Geometry check sheet. Reference: the model listing, model coordinates, mm. Face numbers are marked on the shaded views. A direction names the side the tool comes from. Round coordinates to 2 decimals unless told otherwise and drop trailing zeros. Order: outer loops, then holes, each group sorted by start corner. A loop starts at its lowest first (then second) coordinate and runs counter-clockwise, first axis right, second up. Notation, with made-up numbers: (68.25, -34.75) - (104.25, -34.75) arc R25 ccw to (104.25, -1.75) - close; hole circle Ø1 at (-22.75, -1). An arc over 180 degrees is marked (long way). One line per question, with ' | ' between items. Start each with the question number.
Q1. Sectioned sample at D-D, the plane z = -2.25. Enter the section's corners in (x, y) (3 decimals), then the cut area to 3 significant figures.
Q2. Sectioned sample at C-C, the plane y = 8.75. Enter the section's corners in (x, z).
Q3. Sectioned sample at A-A, the plane z = 4. Enter the section's corners in (x, y) (3 decimals), then the cut area to 3 significant figures.
Q4. Tool access check on the marked faces 1, 2, 3, 4 and 5. Record the directions out of +Z, -Z, +X, -X, +Y, -Y that give a thin tool (end or side, any length) a straight path to the whole face; none if there is none.
Q5. Material ranges on line 1 along Y through (x, z) = (11.1, 1.25) (3 decimals); line 2 along X through (y, z) = (4.5, 1.25); line 3 along X through (y, z) = (3.75, 4.5), recorded low to high.
Q6. Sectioned sample at B-B, the plane x = 11.1. Enter the section's corners in (y, z) (3 decimals).
Q7. Mould release check, pull along X, two halves, no side actions. Record for the marked faces 6, 7 and 8: +X half, -X half, draft (parallel to the pull), parting line (faces both ways), or undercut.
Q8. Gauge pin test, flat ends, axial feed: P1, Ø2.5, axis at y = 4.5, z = -4, coming from the -X side; P2, Ø3, axis at x = 22.5, y = 4, coming from the -Z side; P3, Ø1.3, axis at x = 24.5, z = -7, coming from the +Y side (3 decimals); P4, Ø3, axis at y = 4.5, z = 6, coming from the -X side. Record the tip position at first contact, or that the pin passes through.
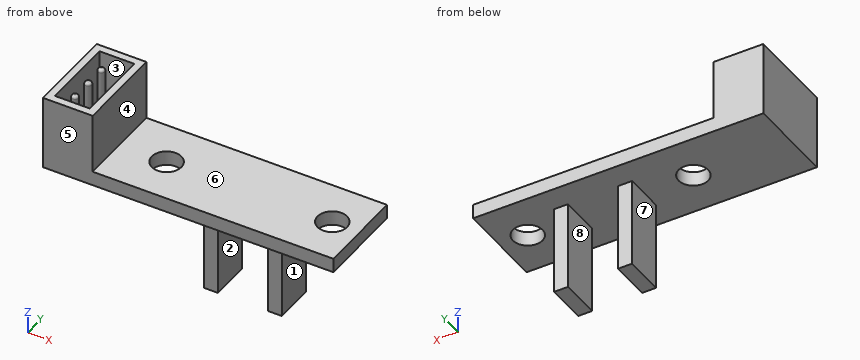
```python
from build123d import *

# Parameters (mm, degrees)
SKETCH_1_W          = 33.3
SKETCH_1_H          = 10.25
EXTRUDE_1_DEPTH     = 1.66
SKETCH_2_W          = 5.7
SKETCH_2_H          = 10.25
EXTRUDE_3_DEPTH     = 6.89
SKETCH_3_W          = 4
SKETCH_3_H          = 8.5
CUT_EXTRUDE_1_DEPTH = 6.05
SKETCH_4_R          = 0.4
EXTRUDE_4_DEPTH     = 5.5
FILLET_1_R          = 0.3
SKETCH_5_R          = 1.7
CUT_EXTRUDE_2_DEPTH = 36.516539809
SKETCH_6_W          = 1.6
SKETCH_6_H          = 4.6
EXTRUDE_5_DEPTH     = 10.19


with BuildPart() as part:
    # Эскиз1 → Бобышка-Вытянуть1 (new body)
    with BuildSketch(Plane.XY):
        with Locations((16.65, 5.125)):
            Rectangle(SKETCH_1_W, SKETCH_1_H)
    extrude(amount=EXTRUDE_1_DEPTH)

    # Эскиз2 → Бобышка-Вытянуть3 (add)
    with BuildSketch(Plane.XY.offset(1.66)):
        with Locations((2.85, 5.125)):
            Rectangle(SKETCH_2_W, SKETCH_2_H)
    extrude(amount=EXTRUDE_3_DEPTH)

    # Эскиз3 → Вырез-Вытянуть1 (cut)
    with BuildSketch(Plane.XY.offset(8.55)):
        with Locations((2.85, 5.125)):
            Rectangle(SKETCH_3_W, SKETCH_3_H)
    extrude(amount=-CUT_EXTRUDE_1_DEPTH, mode=Mode.SUBTRACT)

    # Эскиз4 → Бобышка-Вытянуть4 (add)
    with BuildSketch(Plane.XY.offset(2.5)):
        with Locations((2.050760191, 5.231038637)):
            Circle(SKETCH_4_R)
        with Locations((2.050760191, 7.741038637)):
            Circle(SKETCH_4_R)
        with Locations((2.050760191, 2.721038637)):
            Circle(SKETCH_4_R)
    extrude(amount=EXTRUDE_4_DEPTH)

    # Скругление1
    fillet_1_edges = [part.edges().sort_by_distance(p)[0] for p in [
        (1.650760191, 5.231038637, 8),
        (1.650760191, 7.741038637, 8),
        (1.650760191, 2.721038637, 8),
    ]]
    fillet(fillet_1_edges, radius=FILLET_1_R)

    # Эскиз5 → Вырез-Вытянуть2 (cut, through all)
    with BuildSketch(Plane.XY.offset(1.66)):
        with Locations((11.1, 5.125)):
            Circle(SKETCH_5_R)
        with Locations((30.1, 5.125)):
            Circle(SKETCH_5_R)
    extrude(amount=-CUT_EXTRUDE_2_DEPTH, mode=Mode.SUBTRACT)

    # Эскиз6 → Бобышка-Вытянуть5 (add)
    with BuildSketch(Plane(origin=(0, 0, 0), x_dir=(-1, 0, 0), z_dir=(0, 0, -1))):
        with Locations((-24.9, 5.125)):
            Rectangle(SKETCH_6_W, SKETCH_6_H)
        with Locations((-17.55, 5.125)):
            Rectangle(SKETCH_6_W, SKETCH_6_H)
    extrude(amount=EXTRUDE_5_DEPTH)


solid = part.part
```
Determined:
1) outline: (16.75, 2.825) - (18.35, 2.825) - (18.35, 7.425) - (16.75, 7.425) - close; (24.1, 2.825) - (25.7, 2.825) - (25.7, 7.425) - (24.1, 7.425) - close | area: 14.7 mm2
2) outline: (0, 0) - (33.3, 0) - (33.3, 1.66) - (5.7, 1.66) - (5.7, 8.55) - (4.85, 8.55) - (4.85, 2.5) - (0.85, 2.5) - (0.85, 8.55) - (0, 8.55) - close
3) outline: (0, 0) - (5.7, 0) - (5.7, 10.25) - (0, 10.25) - close; circle Ø0.8 at (2.051, 2.721); circle Ø0.8 at (2.051, 5.231); circle Ø0.8 at (2.051, 7.741); hole (0.85, 0.875) - (4.85, 0.875) - (4.85, 9.375) - (0.85, 9.375) - close | area: 25.9 mm2
4) face 1: -Z, +X, +Y, -Y | face 2: -Z, +Y, -Y | face 3: +Z | face 4: +Z, +X, +Y, -Y | face 5: +Z, -Z, +X, -X, -Y
5) line 1: y = 0 to 3.425, 6.825 to 10.25 | line 2: x = 0 to 9.52, 12.68 to 28.52, 31.68 to 33.3 | line 3: x = 0 to 0.85, 4.85 to 5.7
6) outline: (0, 0) - (3.425, 0) - (3.425, 1.66) - (0, 1.66) - close; (6.825, 0) - (10.25, 0) - (10.25, 1.66) - (6.825, 1.66) - close
7) face 6: draft | face 7: -X half | face 8: undercut
8) P1: stops at x = 16.75 | P2: stops at z = 0 | P3: stops at y = 7.425 | P4: stops at x = 0
